Could you check a few things on this model? Use its own coordinates, in mm. Give positions to 0.01 mm unless a question says otherwise; leave off trailing zeros. Write each loop counter-clockwise with the first axis right and the second up, starting at its lowest first coordinate (ties: lowest second). Pieces come first, ordered by that corner, then holes. Notation, with made-up numbers: (12, 71) - (56, 71) arc R17 cw to (56, 88) - close; hole circle Ø1 at (-7, -27.5). An arc over 180 degrees is marked (long way). Answer as a JSON object with one key per item and string values. Group by question number.
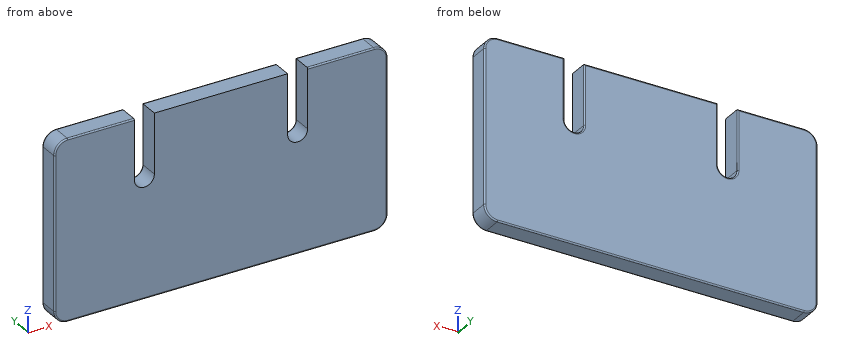
```python
from build123d import *

# Parameters (mm, degrees)
BOSS_EXTRUDE1_DEPTH = 3
FILLET1_R           = 0.2


with BuildPart() as part:
    # Sketch1 → Boss-Extrude1 (new body)
    with BuildSketch(Plane(origin=(0, 0, 0), x_dir=(1, 0, 0), z_dir=(0, 1, 0))):
        with BuildLine():
            Line((10, 0), (-10, 0))
            Line((-10, 0), (-10, 9))
            ThreePointArc((-10, 9), (-11.5, 10.5), (-13, 9))
            Line((-13, 9), (-13, 0))
            Line((-13, 0), (-23, 0))
            ThreePointArc((-23, 0), (-24.414213562, 0.585786438), (-25, 2))
            Line((-25, 2), (-25, 25))
            ThreePointArc((-25, 25), (-24.414213562, 26.414213562), (-23, 27))
            Line((-23, 27), (23, 27))
            ThreePointArc((23, 27), (24.414213562, 26.414213562), (25, 25))
            Line((25, 25), (25, 2))
            ThreePointArc((25, 2), (24.414213562, 0.585786438), (23, 0))
            Line((23, 0), (13, 0))
            Line((13, 0), (13, 9))
            ThreePointArc((13, 9), (11.5, 10.5), (10, 9))
            Line((10, 9), (10, 0))
        make_face()
    extrude(amount=BOSS_EXTRUDE1_DEPTH)

    # Fillet1
    fillet1_edges = [part.edges().sort_by_distance(p)[0] for p in [
        (0, 3, 0),
        (10, 3, -4.5),
        (-18, 0, 0),
        (-24.414213562, 0, -0.585786438),
        (-25, 0, -13.5),
        (-24.414213562, 0, -26.414213562),
        (11.5, 3, -10.5),
        (0, 0, -27),
        (24.414213562, 0, -26.414213562),
        (25, 0, -13.5),
        (24.414213562, 0, -0.585786438),
        (18, 0, 0),
        (13, 3, -4.5),
        (18, 3, 0),
        (24.414213562, 3, -0.585786438),
        (25, 3, -13.5),
        (24.414213562, 3, -26.414213562),
        (0, 3, -27),
        (-24.414213562, 3, -26.414213562),
        (-11.5, 3, -10.5),
        (-25, 3, -13.5),
        (-24.414213562, 3, -0.585786438),
        (-18, 3, 0),
        (-13, 3, -4.5),
        (-10, 3, -4.5),
    ]]
    fillet(fillet1_edges, radius=FILLET1_R)


solid = part.part
```
(1) I want a section at A-A, the plane x = -11.5. Please give me the cut outline in (y, z), and give its area (3 significant figures).
(2) I need wall thicknesses on L1, parallel to X at y = 1.3, z = -4; L2, parallel to X at y = 0.5, z = -9.75; L3, parallel to X at y = 2.85, z = -14.5. Which ranges of each line are inside material? Lowest first, please.
(3) I want a section at B-B, the plane y = 2.25. Please give me the cut outline in (x, z), and give its area (3 significant figures).
(4) I want a section at C-C, the plane z = -9.5. State how many separate pieces and enclosed holes the cut face has, and give its area (3 significant figures).
Entries:
{
 "1": {"outline": "(0, -26.8) arc R0.2 ccw to (0.2, -27) - (2.8, -27) arc R0.2 ccw to (3, -26.8) - (3, -10.7) arc R0.2 ccw to (2.8, -10.5) - (0, -10.5) - close", "area": "49.5 mm^2"},
 "2": {"L1": "-25 to -13, -10 to 10, 13 to 25", "L2": "-25 to -12.8, -10.2 to 10.2, 12.8 to 25", "L3": "-24.99 to 24.99"},
 "3": {"outline": "(-25, -25) arc R2 ccw to (-23, -27) - (23, -27) arc R2 ccw to (25, -25) - (25, -2) arc R2 ccw to (23, 0) - (13, 0) - (13, -9) arc R1.5 cw to (10, -9) - (10, 0) - (-10, 0) - (-10, -9) arc R1.5 cw to (-13, -9) - (-13, 0) - (-23, 0) arc R2 ccw to (-25, -2) - close", "area": "1,290 mm^2"},
 "4": {"separate pieces": "3", "enclosed holes": "0", "area": "133 mm^2"}
}
